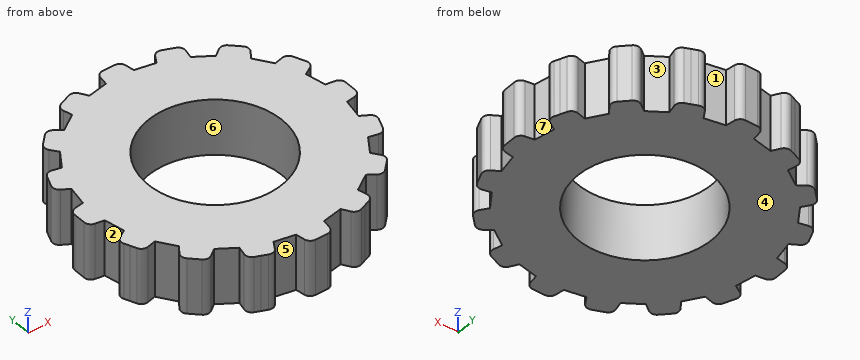
```python
from build123d import *

# Parameters (mm, degrees)
ESQUISSE5_R        = 6
BOSS_EXTRU_1_DEPTH = 5


with BuildPart() as part:
    # Esquisse5 → Boss.-Extru.1 (new body)
    with BuildSketch(Plane.XY):
        with BuildLine():
            Line((0, 12.187189413), (0.508919212, 12.187189413))
            ThreePointArc((0.508919212, 12.187189413), (0.899044051, 12.043043128), (1.101718736, 11.679864778))
            Line((1.101718736, 11.679864778), (1.223875428, 10.898487461))
            Line((1.223875428, 10.898487461), (2.990113971, 10.551498398))
            Line((2.990113971, 10.551498398), (3.397524082, 11.2264814))
            ThreePointArc((3.397524082, 11.2264814), (3.723877023, 11.486437733), (4.140815501, 11.470758379))
            Line((4.140815501, 11.470758379), (4.661933908, 11.254904067))
            Line((4.661933908, 11.254904067), (5.132113951, 11.060149116))
            ThreePointArc((5.132113951, 11.060149116), (5.43737991, 10.777681002), (5.485644567, 10.364587714))
            Line((5.485644567, 10.364587714), (5.29948248, 9.595941861))
            Line((5.29948248, 9.595941861), (6.798487154, 8.59945554))
            Line((6.798487154, 8.59945554), (7.433189829, 9.06714942))
            ThreePointArc((7.433189829, 9.06714942), (7.834181612, 9.182427892), (8.21338231, 9.00838661))
            Line((8.21338231, 9.00838661), (8.612229071, 8.609539849))
            Line((8.612229071, 8.609539849), (8.972089297, 8.249679623))
            ThreePointArc((8.972089297, 8.249679623), (9.146022401, 7.871892888), (9.032529172, 7.47177437))
            Line((9.032529172, 7.47177437), (8.566389797, 6.832879345))
            Line((8.566389797, 6.832879345), (9.569950728, 5.338601775))
            Line((9.569950728, 5.338601775), (10.335318239, 5.52780438))
            ThreePointArc((10.335318239, 5.52780438), (10.749901501, 5.480854889), (11.033634549, 5.174947886))
            Line((11.033634549, 5.174947886), (11.249488861, 4.653829479))
            Line((11.249488861, 4.653829479), (11.444243812, 4.183649436))
            ThreePointArc((11.444243812, 4.183649436), (11.460364322, 3.768058687), (11.202391523, 3.441829356))
            Line((11.202391523, 3.441829356), (10.527240354, 3.029951135))
            Line((10.527240354, 3.029951135), (10.882574489, 1.26537253))
            Line((10.882574489, 1.26537253), (11.662086569, 1.147279478))
            ThreePointArc((11.662086569, 1.147279478), (12.027144767, 0.945249658), (12.172214381, 0.554048503))
            Line((12.172214381, 0.554048503), (12.172214381, -0.010005996))
            Line((12.172214381, -0.010005996), (12.172214381, -0.518925208))
            ThreePointArc((12.172214381, -0.518925208), (12.028068096, -0.909050047), (11.664889747, -1.111724733))
            Line((11.664889747, -1.111724733), (10.88351243, -1.233881424))
            Line((10.88351243, -1.233881424), (10.536523367, -3.000119967))
            Line((10.536523367, -3.000119967), (11.211506369, -3.407530078))
            ThreePointArc((11.211506369, -3.407530078), (11.471462701, -3.733883019), (11.455783348, -4.150821497))
            Line((11.455783348, -4.150821497), (11.239929036, -4.671939904))
            Line((11.239929036, -4.671939904), (11.045174085, -5.142119947))
            ThreePointArc((11.045174085, -5.142119947), (10.76270597, -5.447385906), (10.349612682, -5.495650563))
            Line((10.349612682, -5.495650563), (9.580966829, -5.309488476))
            Line((9.580966829, -5.309488476), (8.584480508, -6.80849315))
            Line((8.584480508, -6.80849315), (9.052174389, -7.443195825))
            ThreePointArc((9.052174389, -7.443195825), (9.167452861, -7.844187609), (8.993411579, -8.223388306))
            Line((8.993411579, -8.223388306), (8.594564817, -8.622235067))
            Line((8.594564817, -8.622235067), (8.234704592, -8.982095293))
            ThreePointArc((8.234704592, -8.982095293), (7.856917857, -9.156028397), (7.456799339, -9.042535168))
            Line((7.456799339, -9.042535168), (6.817904314, -8.576395793))
            Line((6.817904314, -8.576395793), (5.323626744, -9.579956724))
            Line((5.323626744, -9.579956724), (5.512829349, -10.345324235))
            ThreePointArc((5.512829349, -10.345324235), (5.465879858, -10.759907497), (5.159972855, -11.043640545))
            Line((5.159972855, -11.043640545), (4.638854448, -11.259494857))
            Line((4.638854448, -11.259494857), (4.168674404, -11.454249808))
            ThreePointArc((4.168674404, -11.454249808), (3.753083655, -11.470370318), (3.426854324, -11.212397519))
            Line((3.426854324, -11.212397519), (3.014976103, -10.53724635))
            Line((3.014976103, -10.53724635), (1.250397498, -10.892580485))
            Line((1.250397498, -10.892580485), (1.132304447, -11.672092565))
            ThreePointArc((1.132304447, -11.672092565), (0.930274627, -12.037150763), (0.539073472, -12.182220377))
            Line((0.539073472, -12.182220377), (-0.024981027, -12.182220377))
            Line((-0.024981027, -12.182220377), (-0.533900239, -12.182220377))
            ThreePointArc((-0.533900239, -12.182220377), (-0.924025078, -12.038074093), (-1.126699764, -11.674895743))
            Line((-1.126699764, -11.674895743), (-1.248856456, -10.893518426))
            Line((-1.248856456, -10.893518426), (-3.015094998, -10.546529363))
            Line((-3.015094998, -10.546529363), (-3.42250511, -11.221512365))
            ThreePointArc((-3.42250511, -11.221512365), (-3.74885805, -11.481468697), (-4.165796528, -11.465789344))
            Line((-4.165796528, -11.465789344), (-4.686914935, -11.249935032))
            Line((-4.686914935, -11.249935032), (-5.157094979, -11.055180081))
            ThreePointArc((-5.157094979, -11.055180081), (-5.462360938, -10.772711966), (-5.510625594, -10.359618678))
            Line((-5.510625594, -10.359618678), (-5.324463507, -9.590972826))
            Line((-5.324463507, -9.590972826), (-6.823468181, -8.594486504))
            Line((-6.823468181, -8.594486504), (-7.458170856, -9.062180385))
            ThreePointArc((-7.458170856, -9.062180385), (-7.85916264, -9.177458857), (-8.238363337, -9.003417575))
            Line((-8.238363337, -9.003417575), (-8.637210099, -8.604570813))
            Line((-8.637210099, -8.604570813), (-8.997070324, -8.244710588))
            ThreePointArc((-8.997070324, -8.244710588), (-9.171003428, -7.866923853), (-9.057510199, -7.466805335))
            Line((-9.057510199, -7.466805335), (-8.591370824, -6.82791031))
            Line((-8.591370824, -6.82791031), (-9.594931756, -5.33363274))
            Line((-9.594931756, -5.33363274), (-10.360299266, -5.522835345))
            ThreePointArc((-10.360299266, -5.522835345), (-10.774882529, -5.475885854), (-11.058615577, -5.169978851))
            Line((-11.058615577, -5.169978851), (-11.274469888, -4.648860444))
            Line((-11.274469888, -4.648860444), (-11.469224839, -4.178680401))
            ThreePointArc((-11.469224839, -4.178680401), (-11.48534535, -3.763089651), (-11.22737255, -3.43686032))
            Line((-11.22737255, -3.43686032), (-10.552221381, -3.024982099))
            Line((-10.552221381, -3.024982099), (-10.907555516, -1.260403495))
            Line((-10.907555516, -1.260403495), (-11.687067596, -1.142310443))
            ThreePointArc((-11.687067596, -1.142310443), (-12.052125795, -0.940280623), (-12.197195409, -0.549079468))
            Line((-12.197195409, -0.549079468), (-12.197195409, 0.014975031))
            Line((-12.197195409, 0.014975031), (-12.197195409, 0.523894243))
            ThreePointArc((-12.197195409, 0.523894243), (-12.053049124, 0.914019082), (-11.689870774, 1.116693768))
            Line((-11.689870774, 1.116693768), (-10.908493457, 1.238850459))
            Line((-10.908493457, 1.238850459), (-10.561504394, 3.005089002))
            Line((-10.561504394, 3.005089002), (-11.236487396, 3.412499114))
            ThreePointArc((-11.236487396, 3.412499114), (-11.496443729, 3.738852054), (-11.480764375, 4.155790532))
            Line((-11.480764375, 4.155790532), (-11.264910063, 4.676908939))
            Line((-11.264910063, 4.676908939), (-11.070155112, 5.147088983))
            ThreePointArc((-11.070155112, 5.147088983), (-10.787686998, 5.452354942), (-10.37459371, 5.500619598))
            Line((-10.37459371, 5.500619598), (-9.605947857, 5.314457511))
            Line((-9.605947857, 5.314457511), (-8.609461536, 6.813462185))
            Line((-8.609461536, 6.813462185), (-9.077155416, 7.44816486))
            ThreePointArc((-9.077155416, 7.44816486), (-9.192433888, 7.849156644), (-9.018392606, 8.228357341))
            Line((-9.018392606, 8.228357341), (-8.619545845, 8.627204103))
            Line((-8.619545845, 8.627204103), (-8.259685619, 8.987064328))
            ThreePointArc((-8.259685619, 8.987064328), (-7.881898884, 9.160997432), (-7.481780366, 9.047504203))
            Line((-7.481780366, 9.047504203), (-6.842885341, 8.581364828))
            Line((-6.842885341, 8.581364828), (-5.348607771, 9.58492576))
            Line((-5.348607771, 9.58492576), (-5.537810376, 10.35029327))
            ThreePointArc((-5.537810376, 10.35029327), (-5.490860885, 10.764876533), (-5.184953883, 11.04860958))
            Line((-5.184953883, 11.04860958), (-4.663835475, 11.264463892))
            Line((-4.663835475, 11.264463892), (-4.193655432, 11.459218843))
            ThreePointArc((-4.193655432, 11.459218843), (-3.778064683, 11.475339354), (-3.451835352, 11.217366554))
            Line((-3.451835352, 11.217366554), (-3.039957131, 10.542215385))
            Line((-3.039957131, 10.542215385), (-1.275378526, 10.89754952))
            Line((-1.275378526, 10.89754952), (-1.157285475, 11.6770616))
            ThreePointArc((-1.157285475, 11.6770616), (-0.955255654, 12.042119799), (-0.564054499, 12.187189413))
            Line((-0.564054499, 12.187189413), (0, 12.187189413))
        make_face()
        Circle(ESQUISSE5_R, mode=Mode.SUBTRACT)
    extrude(amount=BOSS_EXTRU_1_DEPTH)


solid = part.part
```
Could you check a few things on this model? Use its own coordinates, in mm. Face numbers are marked on the shaded views. A direction names the side the tool comes from. Round coordinates to 2 decimals unless told otherwise and drop trailing zeros. Write each loop counter-clockwise with the first axis right and the second up, starting at its lowest first coordinate (ties: lowest second). Pieces come first, ordered by that corner, then holes.
(1) Which directions (+Z, -Z, +X, -X, +Y, -Y) give clear straight access to the entire face, cutting with the end or side of a thin tool? Please do the marked faces 5, 6 and 7.
Findings below:
face 5: +Z, -Z, -Y
face 6: +Z, -Z
face 7: +Z, -Z, +X
(2) If I drill on probe 1 along Y at (x, z) = (-11, 2.9); probe 2 along Y at (x, z) = (0, 3.1); probe 3 along Y at (x, z) = (-5.25, 1.7), over which ranges is the centre line in solid material (lowest first)?
Findings below:
probe 1: y = -5.28 to -3.3, -1.25 to 1.22, 3.27 to 5.27
probe 2: y = -12.18 to -6, 6 to 12.19
probe 3: y = -11.01 to -2.9, 2.9 to 11.02
(3) Thinking about a two-plate mould opening in X: for the marked faces 1, 2, 3 and 4, which applies, +X half, -X half, draft (parallel to the pull), parting line (faces both ways), or undercut?
Findings below:
face 1: undercut
face 2: -X half
face 3: undercut
face 4: draft
(4) Suppose I cut it at C-C on x = 10. Write out the boundary of the cut face in (y, z), and give its area (3 significant figures).
Findings below:
outline: (-5.41, 0) - (5.44, 0) - (5.44, 5) - (-5.41, 5) - close
area: 54.3 mm2
(5) Suppose I cut it at A-A on x = 0. Write out the boundary of the cut face in (y, z), and give its area (3 significant figures).
Findings below:
outline: (-12.18, 0) - (-6, 0) - (-6, 5) - (-12.18, 5) - close; (6, 0) - (12.19, 0) - (12.19, 5) - (6, 5) - close
area: 61.8 mm2
(6) Suppose I cut it at B-B on y = 3.75. Write out the boundary of the cut face in (x, z).
Findings below:
outline: (-11.5, 0) - (-4.68, 0) - (-4.68, 5) - (-11.5, 5) - close; (4.68, 0) - (11.45, 0) - (11.45, 5) - (4.68, 5) - close
(7) For pin 1 (1 mm diameter, centred on y = -3, z = 4, fed in from +X), with a flat end and sliding along its axis, tell me the tip position at first contact or that it passes through.
Findings below:
pin 1: stops at x = 11.33
